Geometry check sheet. Reference: the model listing, model coordinates, mm. Face numbers are marked on the shaded views. A direction names the side the tool comes from. Coordinates: 2 decimals unless noted, no trailing zeros. Write each loop counter-clockwise with the first axis right and the second up, starting at its lowest first coordinate (ties: lowest second). Pieces come first, ordered by that corner, then holes. Notation, with made-up numbers: M -18.75,0.25 L 5.25,0.25 A25 cw 5.25,27.25 Z; hole C -9,32.5 d5. An arc over 180 degrees is marked long. Put each result on its own line as item: value. Start each with the question number.
1) Gauge pin test, flat ends, axial feed: pin 1 (19.5 mm diameter, centred on x = 134.5, y = -0.5, fed in from -Z); pin 2 (3 mm diameter, centred on y = 7.5, z = 27.5, fed in from -X); pin 3 (4 mm diameter, centred on y = 41.5, z = 7.5, fed in from +X). Record the tip position at first contact, or that the pin passes through.
2) Scan lines: line 1 along Z through (x, y) = (-20.5, 35.5); line 2 along Y through (x, z) = (-52, 17) (3 decimals); line 3 along Z through (x, y) = (-29, -7.5). Record each from-to range of solid material in increasing order.
3) Cross-section at B-B on z = 74.5. Record the cut outline in (x, y), plus the area to 3 significant figures.
4) Set-up check for the marked faces 5, 6 and 7: record each of +Z, -Z, +X, -X, +Y, -Y from which the full face is reachable in a straight line by a thin tool's end or side.
5) Cross-section at A-A on y = 30. Record the cut outline in (x, z), plus the area to 3 significant figures.
6) Mould release check, pull along X, two halves, no side actions. Record for the marked faces 1, 2, 3 and 4: released by +X, released by -X, zero draft, split by the parting line, or undercut.
7) Cross-section at C-C on y = -30.5. Record the cut outline in (x, z).
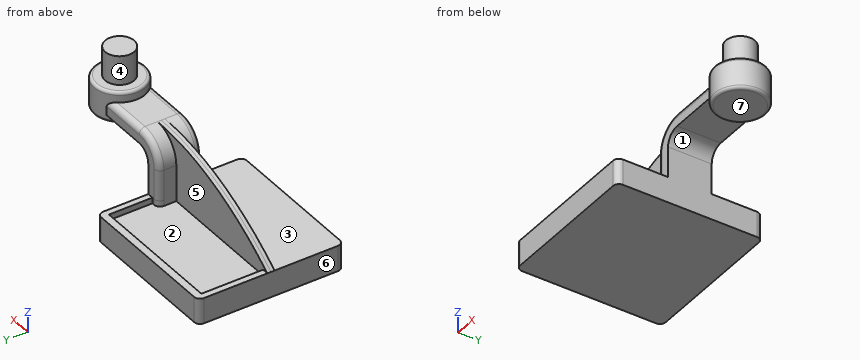
from build123d import *

# Parameters (mm, degrees)
F1_DEPTH  = 63.5
F0_W      = 22.2259311114
F0_H      = 12.7
F2_DEPTH  = 19.05
F3_DEPTH  = 3.175
F5_R      = 5.08
F6_R      = 2.54
F7_R      = 2.54
F8_R      = 12.7
F9_DEPTH  = 25.4
F11_DEPTH = 5.08


with BuildPart() as f1:
    # F0 (on Front) → F1 (new body, symmetric)
    with BuildSketch(Plane.XZ):
        Polygon((52.4926696301, 11.1897839233), (-65.1926696301, 11.1897839233), (-65.1926696301, -11.1897839233), (65.1926696301, -11.1897839233), (65.1926696301, 11.1897839233), align=None)
    extrude(amount=F1_DEPTH, both=True)

    # F0 (on Front) → F2 (join, symmetric)
    with BuildSketch(Plane.XZ):
        with BuildLine():
            Line((52.4926696301, 37.8246089722), (52.4926696301, 11.1897839233))
            Line((52.4926696301, 11.1897839233), (65.1926696301, 11.1897839233))
            Line((65.1926696301, 11.1897839233), (65.1926696301, 37.8246089722))
            ThreePointArc((65.1926696301, 37.8246089722), (68.6156766444, 46.0884789304), (76.8795466026, 49.5114859448))
            Line((76.8795466026, 49.5114859448), (108.1594081487, 49.5114859448))
            Line((108.1594081487, 49.5114859448), (108.1594081487, 62.2114859448))
            Line((108.1594081487, 62.2114859448), (76.8795466026, 62.2114859448))
            ThreePointArc((76.8795466026, 62.2114859448), (59.6354205233, 55.0687350515), (52.4926696301, 37.8246089722))
        make_face()
        with Locations((119.2723737044, 55.8614859448)):
            Rectangle(F0_W, F0_H)
    extrude(amount=F2_DEPTH, both=True)

    # F0 (on Front) → F3 (join, symmetric)
    with BuildSketch(Plane.XZ):
        with BuildLine():
            add(Edge.make_bspline(
                [(-65.1926696301, 11.1897839233), (-26.2716710567, 40.8670417964), (23.8391105086, 62.7601072192), (76.8795466026, 62.2114859448)],
                knots=[0, 0, 0, 0, 150.9560489097, 150.9560489097, 150.9560489097, 150.9560489097], degree=3))
            Line((-65.1926696301, 11.1897839233), (52.4926696301, 11.1897839233))
            Line((52.4926696301, 11.1897839233), (52.4926696301, 37.8246089722))
            ThreePointArc((52.4926696301, 37.8246089722), (59.6354205233, 55.0687350515), (76.8795466026, 62.2114859448))
        make_face()
        with Locations((119.2723737044, 55.8614859448)):
            Rectangle(F0_W, F0_H)
    extrude(amount=F3_DEPTH, both=True)

    # F0 (on Front) → F4 (revolve)
    with BuildSketch(Plane.XZ):
        Polygon((130.3853392601, 71.0308142006), (130.3853392601, 62.2114859448), (130.3853392601, 49.5114859448), (130.3853392601, 43.7861196697), (152.6112703715, 43.7861196697), (152.6112703715, 71.0308142006), align=None)
    revolve(axis=Axis((130.3853392601, 0, 57.4084669352), (0, 0, -1)))

    # F5
    f5_edges = [f1.edges().sort_by_distance(p)[0] for p in [
        (-65.19267, -63.5, 0),
        (65.19267, -63.5, 0),
        (65.19267, 63.5, 0),
        (-65.19267, 63.5, 0),
        (52.49267, 19.05, 24.507196),
        (52.49267, -19.05, 24.507196),
    ]]
    fillet(f5_edges, radius=F5_R)

    # F6
    f6_edges = [f1.edges().sort_by_distance(p)[0] for p in [
        (108.159408, 0, 71.030814),
    ]]
    fillet(f6_edges, radius=F6_R)

    # F7
    f7_edges = [f1.edges().sort_by_distance(p)[0] for p in [
        (108.159408, 0, 43.78612),
    ]]
    fillet(f7_edges, radius=F7_R)

    # F8 (on face) → F9 (join)
    with BuildSketch(Plane.XY.offset(71.0308142006)):
        with Locations((130.3853392601, 0)):
            Circle(F8_R)
    extrude(amount=F9_DEPTH)

    # F10 (on face) → F11 (cut)
    with BuildSketch(Plane.XY.offset(11.1897839233)):
        with BuildLine():
            Line((59.8586685956, 56.9533742964), (-59.6454292536, 56.9533742964))
            Line((-59.6454292536, 56.9533742964), (-59.6454292536, 3.175))
            Line((-59.6454292536, 3.175), (52.4926696301, 3.175))
            Line((52.4926696301, 3.175), (52.4926696301, 13.97))
            ThreePointArc((52.4926696301, 13.97), (53.9805671816, 17.5621024484), (57.5726696301, 19.05))
            Line((57.5726696301, 19.05), (59.8586685956, 19.05))
            Line((59.8586685956, 19.05), (59.8586685956, 56.9533742964))
        make_face()
    extrude(amount=-F11_DEPTH, mode=Mode.SUBTRACT)


solid = f1.part
Answer key:
1. pin 1: stops at z = 43.79
1. pin 2: stops at x = 52.49
1. pin 3: stops at x = 65.19
2. line 1: z = -11.19 to 6.11
2. line 2: y = -3.175 to 3.175
2. line 3: z = -11.19 to 11.19
3. outline: C 130.39,0 d25.4
3. area: 507 mm²
4. face 5: +Z
4. face 6: +Z, -Z, -X, +Y, -Y
4. face 7: -Z, +X, +Y, -Y
5. outline: M -65.19,-11.19 L 65.19,-11.19 L 65.19,11.19 L 59.86,11.19 L 59.86,6.11 L -59.65,6.11 L -59.65,11.19 L -65.19,11.19 Z
5. area: 2,310 mm²
6. face 1: undercut
6. face 2: undercut
6. face 3: zero draft
6. face 4: split by the parting line
7. outline: M -65.19,-11.19 L 65.19,-11.19 L 65.19,11.19 L -65.19,11.19 Z
